Could you check a few things on this drawing? It's one solid part, dimensions in mm from its lowest x, y, z. Give positions to 0.01 mm unless a question says otherwise; leave off trailing zeros. Order: outer loops, then holes, each group sorted by start corner. A loop starts at its lowest first (then second) coordinate and runs counter-clockwise, first axis right, second up. Notation, with made-up numbers: (59, 50) -> (86, 50) arc R17 cw to (86, 76) -> close; hole circle Ø11 at (84.5, 57.25). An arc over 180 degrees is marked (long way). Answer as a JSON object with one key per item and string values.
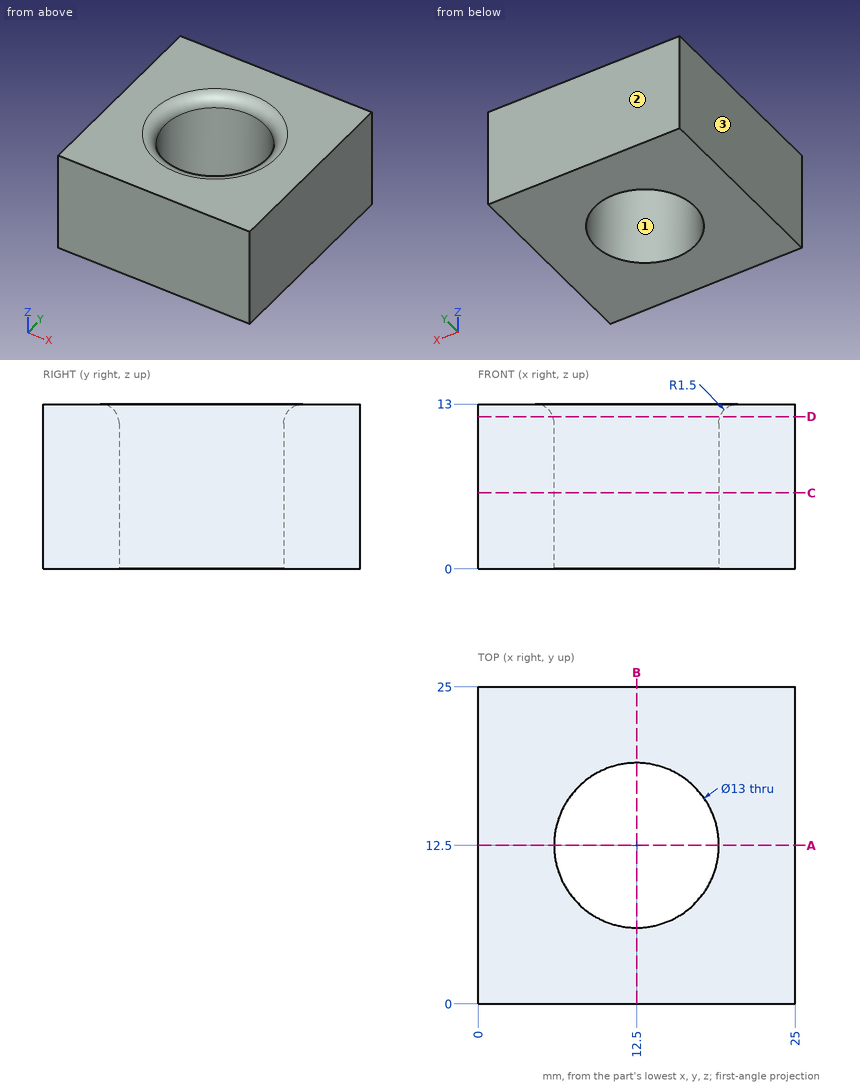
1. Please list where these lines run through material, in increasing order: L1, parallel to Y at x = 12.5, z = 5.75; L2, parallel to Y at x = 18, z = 7.
Worked answers:
{"L1": "0 to 6, 19 to 25", "L2": "0 to 9.04, 15.96 to 25"}
2. If we section it at A-A on y = 12.5: Please give me the cut outline in (x, z).
Worked answers:
{"outline": "(0, 0) -> (6, 0) -> (6, 11.5) arc R1.5 ccw to (4.5, 13) -> (0, 13) -> close; (19, 0) -> (25, 0) -> (25, 13) -> (20.5, 13) arc R1.5 ccw to (19, 11.5) -> close"}
3. If we mould it in two halves opening along Y, with no side actions, what happens to the marked faces 1, 2 and 3? For each: +Y half, -Y half, draft (parallel to the pull), parting line (faces both ways), or undercut.
Worked answers:
{"face 1": "undercut", "face 2": "+Y half", "face 3": "draft"}
4. If we section it at C-C on z = 6: Please give me the cut outline in (x, y).
Worked answers:
{"outline": "(0, 0) -> (25, 0) -> (25, 25) -> (0, 25) -> close; hole circle Ø13 at (12.5, 12.5)"}
5. Will these pins go through, and if not, where does the flat tip stop? pin 1 Ø5 at (x, y) = (15, 17) entering from +Z; pin 2 Ø1.5 at (x, y) = (22, 8.5) entering from -Z.
Worked answers:
{"pin 1": "z = 12.96", "pin 2": "z = 0"}
6. If we section it at D-D on z = 12: Please give me the cut outline in (x, y), then the cut area to 3 significant figures.
Worked answers:
{"outline": "(0, 0) -> (25, 0) -> (25, 25) -> (0, 25) -> close; hole circle Ø13.17 at (12.5, 12.5)", "area": "489 mm²"}
